from build123d import *

# Parameters (mm, degrees)
BOSS_EXTRUDE1_DEPTH      = 2.5
SKETCH2_W                = 20
SKETCH2_H                = 12
CUT_EXTRUDE1_DEPTH       = 3
BOSS_EXTRUDE3_DEPTH      = 6
BOSS_EXTRUDE3_DEPTH_BACK = 5
BOSS_EXTRUDE4_DEPTH      = 20
BOSS_EXTRUDE5_DEPTH      = 20
SKETCH14_R               = 1.5
CUT_EXTRUDE6_DEPTH       = 178
SKETCH11_W               = 27
SKETCH11_H               = 3
CUT_EXTRUDE7_DEPTH       = 10
SKETCH15_R               = 1.25
SKETCH15_W               = 120
SKETCH15_H               = 20
CUT_EXTRUDE8_DEPTH       = 12
SKETCH15_3_R             = 1.25
SKETCH15_3_W             = 120
SKETCH15_3_H             = 20
CUT_EXTRUDE9_DEPTH       = 4
SKETCH17_W               = 30
SKETCH17_H               = 22
BOSS_EXTRUDE6_DEPTH      = 7
SKETCH18_W               = 12
SKETCH18_H               = 6
CUT_EXTRUDE11_DEPTH      = 30
SKETCH19_W               = 12
SKETCH19_H               = 6
CUT_EXTRUDE12_DEPTH      = 30
SKETCH16_W               = 85
SKETCH16_H               = 70
CUT_EXTRUDE13_DEPTH      = 2
SKETCH20_R               = 19.5
BOSS_EXTRUDE7_DEPTH      = 13.7
FILLET1_R                = 10
FILLET2_R                = 5
SKETCH21_W               = 30
SKETCH21_H               = 22
BOSS_EXTRUDE8_DEPTH      = 5


with BuildPart() as part:
    # Sketch1 → Boss-Extrude1 (new body, symmetric)
    with BuildSketch(Plane(origin=(0, 0, 0), x_dir=(1, 0, 0), z_dir=(0, 1, 0))):
        with BuildLine():
            Line((-21, 56.5), (-21, 26.5))
            Line((-21, 26.5), (-55, 8.5))
            Line((-55, 8.5), (-55, -69.5))
            Line((-55, -69.5), (-60, -69.5))
            Line((-60, -69.5), (-60, -91.5))
            Line((-60, -91.5), (60, -91.5))
            Line((60, -91.5), (60, -69.5))
            Line((60, -69.5), (55, -69.5))
            Line((55, -69.5), (55, 8.5))
            Line((55, 8.5), (21, 26.5))
            Line((21, 26.5), (21, 56.5))
            Line((21, 56.5), (60, 56.5))
            ThreePointArc((60, 56.5), (63.535533906, 57.964466094), (65, 61.5))
            Line((65, 61.5), (65, 86.5))
            ThreePointArc((65, 86.5), (63.535533906, 90.035533906), (60, 91.5))
            Line((60, 91.5), (-60, 91.5))
            ThreePointArc((-60, 91.5), (-63.535533906, 90.035533906), (-65, 86.5))
            Line((-65, 86.5), (-65, 61.5))
            ThreePointArc((-65, 61.5), (-63.535533906, 57.964466094), (-60, 56.5))
            Line((-60, 56.5), (-21, 56.5))
        make_face()
    extrude(amount=BOSS_EXTRUDE1_DEPTH, both=True)

    # Sketch2 → Cut-Extrude1 (cut)
    with BuildSketch(Plane.XZ.offset(2.5)):
        with Locations((-50, 80.5)):
            Rectangle(SKETCH2_W, SKETCH2_H)
        with Locations((50, 80.5)):
            Rectangle(SKETCH2_W, SKETCH2_H)
    extrude(amount=-CUT_EXTRUDE1_DEPTH, mode=Mode.SUBTRACT)

    # Sketch5 → Boss-Extrude3 (add, two sides)
    with BuildSketch(Plane(origin=(0, 2.5, 0), x_dir=(1, 0, 0), z_dir=(0, 1, 0))) as boss_extrude3_sk:
        with BuildLine():
            Line((-60, 56.5), (-60, 54.5))
            ThreePointArc((-60, 54.5), (-64.949747468, 56.550252532), (-67, 61.5))
            Line((-67, 61.5), (-67, 86.5))
            ThreePointArc((-67, 86.5), (-64.949747468, 91.449747468), (-60, 93.5))
            Line((-60, 93.5), (60, 93.5))
            ThreePointArc((60, 93.5), (64.949747468, 91.449747468), (67, 86.5))
            Line((67, 86.5), (67, 61.5))
            ThreePointArc((67, 61.5), (64.949747468, 56.550252532), (60, 54.5))
            Line((60, 54.5), (60, 56.5))
            ThreePointArc((60, 56.5), (63.535533906, 57.964466094), (65, 61.5))
            Line((65, 61.5), (65, 86.5))
            ThreePointArc((65, 86.5), (63.535533906, 90.035533906), (60, 91.5))
            Line((60, 91.5), (-60, 91.5))
            ThreePointArc((-60, 91.5), (-63.535533906, 90.035533906), (-65, 86.5))
            Line((-65, 86.5), (-65, 61.5))
            ThreePointArc((-65, 61.5), (-63.535533906, 57.964466094), (-60, 56.5))
        make_face()
    extrude(amount=BOSS_EXTRUDE3_DEPTH)
    extrude(boss_extrude3_sk.sketch, amount=-BOSS_EXTRUDE3_DEPTH_BACK)

    # Sketch12 → Boss-Extrude4 (add)
    with BuildSketch(Plane.ZY.offset(60)):
        Polygon((74.5, -2.5), (74.5, -4.5), (79.5, -4.5), (79.5, -11.5), (77.5, -11.5), (77.5, -6.5), (72.5, -6.5), (72.5, -4.5), (72.5, -2.5), align=None)
        Polygon((81.5, -11.5), (83.5, -11.5), (83.5, -6.5), (88.5, -6.5), (88.5, -4.5), (88.5, -2.5), (86.5, -2.5), (86.5, -4.5), (81.5, -4.5), align=None)
    extrude(amount=-BOSS_EXTRUDE4_DEPTH)

    # Sketch13 → Boss-Extrude5 (add)
    with BuildSketch(Plane(origin=(60, 0, 0), x_dir=(0, 0, -1), z_dir=(1, 0, 0))):
        Polygon((-86.5, -2.5), (-86.5, -4.5), (-81.5, -4.5), (-81.5, -11.5), (-83.5, -11.5), (-83.5, -6.5), (-88.5, -6.5), (-88.5, -2.5), align=None)
        Polygon((-79.5, -11.5), (-77.5, -11.5), (-77.5, -6.5), (-72.5, -6.5), (-72.5, -2.5), (-74.5, -2.5), (-74.5, -4.5), (-79.5, -4.5), align=None)
    extrude(amount=-BOSS_EXTRUDE5_DEPTH)

    # Sketch14 → Cut-Extrude6 (cut, through all)
    with BuildSketch(Plane.XY.offset(83.5)):
        with Locations((45, -8.5)):
            Circle(SKETCH14_R)
        with Locations((55, -8.5)):
            Circle(SKETCH14_R)
        with Locations((-55, -8.5)):
            Circle(SKETCH14_R)
        with Locations((-45, -8.5)):
            Circle(SKETCH14_R)
    extrude(amount=-CUT_EXTRUDE6_DEPTH, mode=Mode.SUBTRACT)

    # Sketch11 → Cut-Extrude7 (cut)
    with BuildSketch(Plane(origin=(0, 0, -93.5), x_dir=(-1, 0, 0), z_dir=(0, 0, -1))):
        with Locations((0, 4)):
            Rectangle(SKETCH11_W, SKETCH11_H)
    extrude(amount=-CUT_EXTRUDE7_DEPTH, mode=Mode.SUBTRACT)

    # Sketch15 → Cut-Extrude8 (cut, through all)
    with BuildSketch(Plane.XZ.offset(2.5)):
        with Locations((-61.5, -65)):
            Circle(SKETCH15_R)
        with Locations((61.5, -65)):
            Circle(SKETCH15_R)
        with Locations((61.5, -86)):
            Circle(SKETCH15_R)
        with Locations((-61.5, -86)):
            Circle(SKETCH15_R)
        with Locations((0, -75.5)):
            Rectangle(SKETCH15_W, SKETCH15_H)
    extrude(amount=-CUT_EXTRUDE8_DEPTH, mode=Mode.SUBTRACT)

    # Sketch15_3 → Cut-Extrude9 (cut)
    with BuildSketch(Plane.XZ.offset(2.5)):
        with BuildLine():
            Line((-63, -61.5), (63, -61.5))
            ThreePointArc((63, -61.5), (64.414213562, -62.085786438), (65, -63.5))
            Line((65, -63.5), (65, -87.5))
            ThreePointArc((65, -87.5), (64.414213562, -88.914213562), (63, -89.5))
            Line((63, -89.5), (-63, -89.5))
            ThreePointArc((-63, -89.5), (-64.414213562, -88.914213562), (-65, -87.5))
            Line((-65, -87.5), (-65, -63.5))
            ThreePointArc((-65, -63.5), (-64.414213562, -62.085786438), (-63, -61.5))
        make_face()
        with Locations((61.5, -65)):
            Circle(SKETCH15_3_R, mode=Mode.SUBTRACT)
        with Locations((-61.5, -65)):
            Circle(SKETCH15_3_R, mode=Mode.SUBTRACT)
        with Locations((61.5, -86)):
            Circle(SKETCH15_3_R, mode=Mode.SUBTRACT)
        with Locations((-61.5, -86)):
            Circle(SKETCH15_3_R, mode=Mode.SUBTRACT)
        with Locations((0, -75.5)):
            Rectangle(SKETCH15_3_W, SKETCH15_3_H, mode=Mode.SUBTRACT)
    extrude(amount=-CUT_EXTRUDE9_DEPTH, mode=Mode.SUBTRACT)

    # Sketch17 → Boss-Extrude6 (add)
    with BuildSketch(Plane(origin=(0, 2.5, 0), x_dir=(1, 0, 0), z_dir=(0, 1, 0))):
        with Locations((-45, -80.5)):
            Rectangle(SKETCH17_W, SKETCH17_H)
        with Locations((45, -80.5)):
            Rectangle(SKETCH17_W, SKETCH17_H)
    extrude(amount=BOSS_EXTRUDE6_DEPTH)

    # Sketch18 → Cut-Extrude11 (cut)
    with BuildSketch(Plane(origin=(60, 0, 0), x_dir=(0, 0, -1), z_dir=(1, 0, 0))):
        with Locations((-80.5, 3.5)):
            Rectangle(SKETCH18_W, SKETCH18_H)
    extrude(amount=-CUT_EXTRUDE11_DEPTH, mode=Mode.SUBTRACT)

    # Sketch19 → Cut-Extrude12 (cut)
    with BuildSketch(Plane.ZY.offset(60)):
        with Locations((80.5, 3.5)):
            Rectangle(SKETCH19_W, SKETCH19_H)
    extrude(amount=-CUT_EXTRUDE12_DEPTH, mode=Mode.SUBTRACT)

    # Sketch16 → Cut-Extrude13 (cut)
    with BuildSketch(Plane(origin=(0, 2.5, 0), x_dir=(1, 0, 0), z_dir=(0, 1, 0))):
        with Locations((0, -29.5)):
            Rectangle(SKETCH16_W, SKETCH16_H)
    extrude(amount=-CUT_EXTRUDE13_DEPTH, mode=Mode.SUBTRACT)

    # Sketch20 → Boss-Extrude7 (add)
    with BuildSketch(Plane.XZ.offset(2.5)):
        with Locations((0, -41.5)):
            Circle(SKETCH20_R)
    extrude(amount=-BOSS_EXTRUDE7_DEPTH)

    # Fillet1
    fillet1_edges = [part.edges().sort_by_distance(p)[0] for p in [
        (21, 0, -26.5),
        (55, 0, -8.5),
        (-55, 0, -8.5),
        (-21, 0, -26.5),
    ]]
    fillet(fillet1_edges, radius=FILLET1_R)

    # Fillet2
    fillet2_edges = [part.edges().sort_by_distance(p)[0] for p in [
        (21, 0, -56.5),
        (-21, 0, -56.5),
    ]]
    fillet(fillet2_edges, radius=FILLET2_R)

    # Sketch21 → Boss-Extrude8 (add)
    with BuildSketch(Plane(origin=(0, 9.5, 0), x_dir=(1, 0, 0), z_dir=(0, 1, 0))):
        with Locations((45, -80.5)):
            Rectangle(SKETCH21_W, SKETCH21_H)
        with Locations((-45, -80.5)):
            Rectangle(SKETCH21_W, SKETCH21_H)
    extrude(amount=BOSS_EXTRUDE8_DEPTH)


solid = part.part
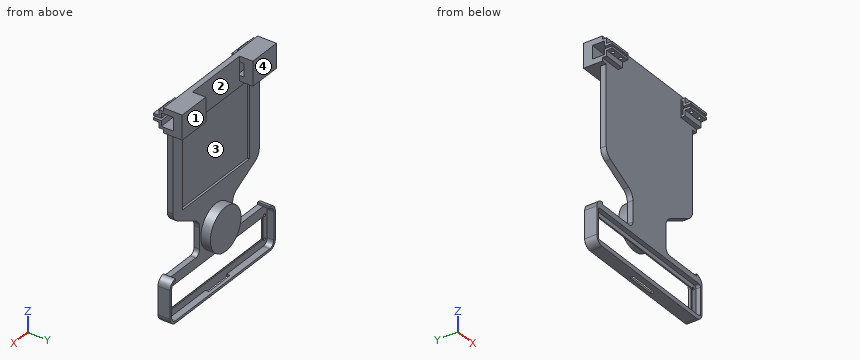
CAD build for the part. Positions are in the model's coordinates, mm. Face numbers are marked on the shaded views. A direction names the side the tool comes from. Give positions to 0.01 mm unless a question says otherwise; leave off trailing zeros. Loops run counter-clockwise (first coordinate to the right, second up) from the corner with the lowest first, then second, coordinate; pieces in that order, holes last. Notation, with made-up numbers: M -11,-22.5 L 41,-22.5 A29 cw 41,3.5 Z; hole C -2,-25 d11. An arc over 180 degrees is marked long. One line per question, with ' | ' between items. Start each with the question number.
1. Saw through at A-A on x = 0. Give the cut face in (y, z), plus the area to 3 significant figures.
2. Probe L1, parallel to Y at x = 45, z = 78.4; L2, parallel to X at y = 1.85, z = -86; L3, parallel to Z at x = -61.5, y = 2.1. List the from-to ranges inside material, lowest first. Write a range as from..to.
3. 3-axis set-ups, long thin cutter, end or side, ignore diameter. For the marked faces 3 and 4: which of +Z, -Z, +X, -X, +Y, -Y reach the whole face in a straight line?
4. Two-plate mould, pull along X, no slides. Class the marked faces 1 and 2: pulls with the +X half, pulls with the -X half, needs draft (parallel to the pull), parting line crosses it, or undercut.
5. Flat gauge pins, fed straight in: pin 1 (0.6 mm diameter, centred on y = 1.5, z = 46, fed in from +X); pin 2 (2.5 mm diameter, centred on x = 52, y = -8.5, fed in from +Z); pin 3 (5 mm diameter, centred on x = 35, z = 28, fed in from +Y). Where does each tip first touch, or does it go through?
6. Saw through at B-B on z = -45. Give the cut face in (x, y).
Result sheet:
1) outline: M -2.5,-93.5 L 2.5,-93.5 L 2.5,-85.5 L 1.5,-85.5 L 1.5,-89.5 L -2.5,-89.5 Z; M -2.5,-61.5 L 1.5,-61.5 L 1.5,-65.5 L 2.5,-65.5 L 2.5,-61 L 11.2,-61 L 11.2,-22 L 2.5,-22 L 2.5,-5.5 L 0.5,-5.5 L 0.5,64.5 L 2.5,64.5 L 2.5,91.5 L -2.5,91.5 Z; M 5.5,-93.5 L 8.5,-93.5 L 8.5,-91.5 L 5.5,-91.5 Z | area: 998 mm^2
2) L1: y = -11.5..-10, -7..-4.5, 6.5..14.5 | L2: x = -67..-62.75, -60.25..60.25, 62.75..67 | L3: z = -93.34..-87.25, -84.75..-66.25, -63.75..-54.66
3) face 3: +Y | face 4: +Z, -Z, +X, -X, +Y
4) face 1: needs draft | face 2: undercut
5) pin 1: stops at x = 55 | pin 2: stops at z = 83.5 | pin 3: stops at y = 0.5
6) outline: M -21,-2.5 L 21,-2.5 L 21,2.5 L 19.18,2.5 L 19.18,11.2 L -19.18,11.2 L -19.18,2.5 L -21,2.5 Z
